from build123d import *

# Parameters (mm, degrees)
ESQUISSE1_W             = 188
ESQUISSE1_H             = 60
BOSS_EXTRU_1_DEPTH      = 6
ESQUISSE3_W             = 50
ESQUISSE3_H             = 52
ENL_V_MAT_EXTRU_2_DEPTH = 10
ESQUISSE6_W             = 6
ESQUISSE6_H             = 20
BOSS_EXTRU_2_DEPTH      = 6
ESQUISSE7_W             = 25
ESQUISSE7_H             = 6
BOSS_EXTRU_3_DEPTH      = 6
ESQUISSE8_R             = 1
ENL_V_MAT_EXTRU_4_DEPTH = 10
ESQUISSE9_W             = 28.5
ESQUISSE9_H             = 6
ESQUISSE9_W_2           = 28
ESQUISSE9_W_3           = 31.5
ENL_V_MAT_EXTRU_5_DEPTH = 10


with BuildPart() as part:
    # Esquisse1 → Boss.-Extru.1 (new body)
    with BuildSketch(Plane.XY):
        Rectangle(ESQUISSE1_W, ESQUISSE1_H)
    extrude(amount=BOSS_EXTRU_1_DEPTH)

    # Esquisse3 → Enlèv. mat.-Extru.2 (cut)
    with BuildSketch(Plane(origin=(0, 0, 0), x_dir=(-1, 0, 0), z_dir=(0, 0, -1))):
        with Locations((69, -4)):
            Rectangle(ESQUISSE3_W, ESQUISSE3_H)
    extrude(amount=-ENL_V_MAT_EXTRU_2_DEPTH, mode=Mode.SUBTRACT)

    # Esquisse6 → Boss.-Extru.2 (add)
    with BuildSketch(Plane(origin=(94, 0, 0), x_dir=(0, 0, -1), z_dir=(1, 0, 0))):
        with Locations((-3, 0)):
            Rectangle(ESQUISSE6_W, ESQUISSE6_H)
    extrude(amount=BOSS_EXTRU_2_DEPTH)

    # Esquisse7 → Boss.-Extru.3 (add)
    with BuildSketch(Plane(origin=(0, 30, 0), x_dir=(1, 0, 0), z_dir=(0, 1, 0))):
        with Locations((53, -3)):
            Rectangle(ESQUISSE7_W, ESQUISSE7_H)
        with Locations((0, -3)):
            Rectangle(ESQUISSE7_W, ESQUISSE7_H)
        with Locations((-53, -3)):
            Rectangle(ESQUISSE7_W, ESQUISSE7_H)
    extrude(amount=BOSS_EXTRU_3_DEPTH)

    # Esquisse8 → Enlèv. mat.-Extru.4 (cut)
    with BuildSketch(Plane(origin=(0, 0, 0), x_dir=(-1, 0, 0), z_dir=(0, 0, -1))):
        with Locations((29, 0)):
            Circle(ESQUISSE8_R)
        with Locations((-4, 0)):
            Circle(ESQUISSE8_R)
    extrude(amount=-ENL_V_MAT_EXTRU_4_DEPTH, mode=Mode.SUBTRACT)

    # Esquisse9 → Enlèv. mat.-Extru.5 (cut)
    with BuildSketch(Plane(origin=(0, 0, 0), x_dir=(-1, 0, 0), z_dir=(0, 0, -1))):
        with Locations((-79.75, -27)):
            Rectangle(ESQUISSE9_W, ESQUISSE9_H)
        with Locations((-26.5, -27)):
            Rectangle(ESQUISSE9_W_2, ESQUISSE9_H)
        with Locations((28.25, -27)):
            Rectangle(ESQUISSE9_W_3, ESQUISSE9_H)
    extrude(amount=-ENL_V_MAT_EXTRU_5_DEPTH, mode=Mode.SUBTRACT)


solid = part.part
Design review of the part built by this model. Coordinates are the model's own, in mm. A direction names the side the tool comes from. Coordinates: 2 decimals unless noted, no trailing zeros. Loops run counter-clockwise (first coordinate to the right, second up) from the corner with the lowest first, then second, coordinate; pieces in that order, holes last.
Item 1: Add section B-B (x = -73). Write out the cut boundary in (y, z), and give its area (3 significant figures).
Completed:
outline: (22, 0) - (30, 0) - (30, 6) - (22, 6) - close
area: 48.0 mm2
Item 2: Wall thickness on L1, parallel to X at y = 32.5, z = 5.4; L2, parallel to Y at x = -29, z = 4.7; L3, parallel to Y at x = 4, z = 4.35: over which ranges is each line inside the solid? List them lowest first.
Completed:
L1: x = -65.5 to -40.5, -12.5 to 12.5, 40.5 to 65.5
L2: y = -24 to -1, 1 to 30
L3: y = -30 to -1, 1 to 36
Item 3: Clearance check with flat-ended pins moving along their axes: pin 1 (1.8 mm diameter, centred on y = -26.5, z = 3, fed in from -X); pin 2 (1.8 mm diameter, centred on y = 32.5, z = 2, fed in from +X); pin 3 (3 mm diameter, centred on y = 32.5, z = 4, fed in from -X). State where each tip first meets the part, or that it passes through.
Completed:
pin 1: stops at x = -12.5
pin 2: stops at x = 65.5
pin 3: stops at x = -65.5
Item 4: Add section A-A (z = 2.15). Give the number of separate pieces and of enclosed holes in the cut face, and give its area (3 significant figures).
Completed:
separate pieces: 1
enclosed holes: 2
area: 8,720 mm2
Item 5: Draft analysis for pull direction X (two halves, no side actions). For faces 1 (the flat face through (-69, 22, 3)), 2 (the flat face through (-12.5, -27, 3)), 3 (the flat face through (40.5, 33, 3)), state which applies: pulls with the +X half, pulls with the -X half, needs draft (parallel to the pull), parting line crosses it, or undercut.
Completed:
face 1: needs draft
face 2: pulls with the -X half
face 3: undercut
Item 6: For faces 4 (the flat face through (27, -24, 3)), 5 (the flat face through (26, 30, 3)), 6 (the flat face through (-28, -24, 3)), 7 (the flat face through (80, 30, 3)), 8 (the flat face through (97, -10, 3)), list the 3-axis set-ups (+Z, -Z, +X, -X, +Y, -Y) from which the entire face can be reached by the end or side of a thin tool; tool diameter is ignored.
Completed:
face 4: +Z, -Z, -Y
face 5: +Z, -Z, +Y
face 6: +Z, -Z, -X, -Y
face 7: +Z, -Z, +X, +Y
face 8: +Z, -Z, +X, -Y
Item 7: Add section C-C (y = -18). Write out the cut boundary in (x, z).
Completed:
outline: (-44, 0) - (94, 0) - (94, 6) - (-44, 6) - close
